Job drawing, mm, ordinate dimensions from the low corner. One solid piece. A direction names the side the tool comes from. Give positions to 0.01 mm unless a question says otherwise; leave off trailing zeros. Order: outer loops, then holes, each group sorted by start corner. A loop starts at its lowest first (then second) coordinate and runs counter-clockwise, first axis right, second up.
1. Drop flat-ended pins along their axis: pin 1 Ø3 at (x, y) = (8.5, 8.5) entering from -Z; pin 2 Ø3 at (y, z) = (15, 0.5) entering from +X; pin 3 Ø1.5 at (x, z) = (13, 0.5) entering from -Y. Give the stop position or say it passes through.
2. Probe line 1 (Y direction, x = 8.5, z = 1.25); line 2 (Z direction, x = 8.25, y = 2.75); line 3 (X direction, y = 7.75, z = 2.05). List the from-to ranges inside material, lowest first.
3. Mould opens along Y. For the marked faces 3, 4 and 5 say: +Y half, -Y half, draft (parallel to the pull), parting line (faces both ways), or undercut.
4. Which spindle directions (+Z, -Z, +X, -X, +Y, -Y) get a long thin tool onto all of the face, cutting with end or side? Do the marked faces 1 and 2. Say none if no direction does.
5. Slice it at D-D on x = 3. List the corners of the cut face in (y, z), and give its area (3 significant figures).
6. Slice it at A-A on y = 8.5. List the corners of the cut face in (x, z), and give its area (3 significant figures).
7. Slice it at C-C on y = 11.5. List the corners of the cut face in (x, z), and give its area (3 significant figures).
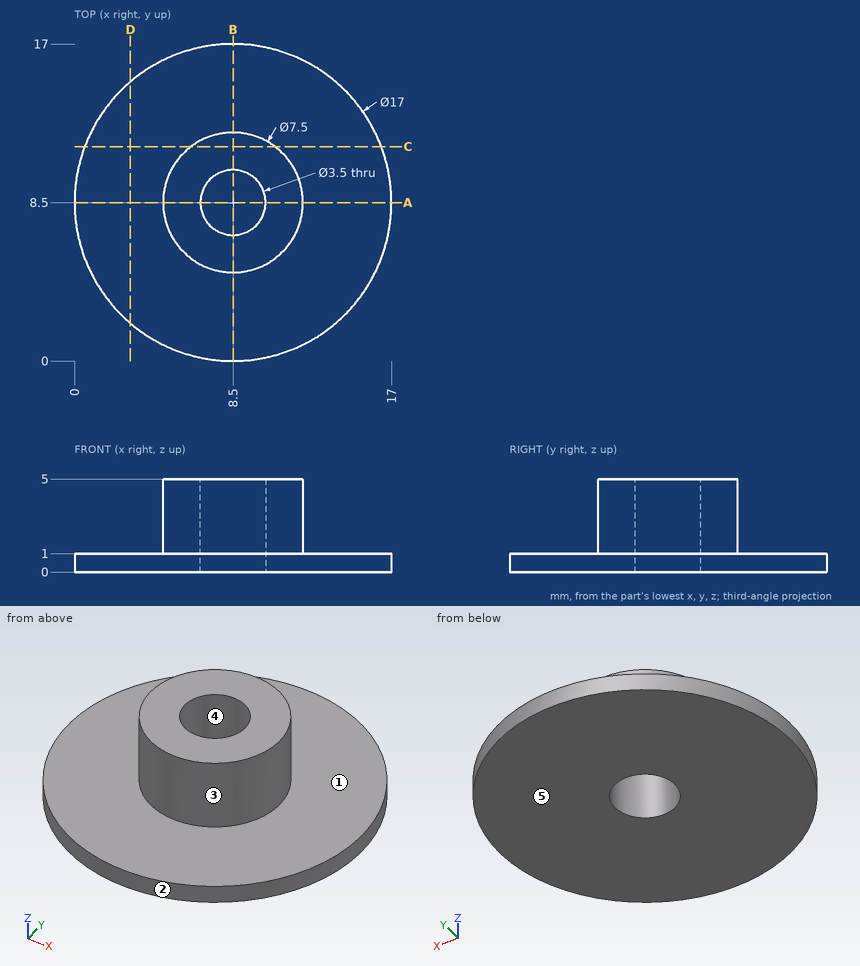
Data:
1. pin 1: passes through
1. pin 2: stops at x = 15.37
1. pin 3: stops at y = 0.87
2. line 1: y = 4.75 to 6.75, 10.25 to 12.25
2. line 2: z = 0 to 1
2. line 3: x = 4.83 to 6.92, 10.08 to 12.17
3. face 3: parting line
3. face 4: undercut
3. face 5: draft
4. face 1: +Z
4. face 2: +Z, -Z
5. outline: (2.02, 0) - (14.98, 0) - (14.98, 1) - (2.02, 1) - close
5. area: 13.0 mm2
6. outline: (0, 0) - (6.75, 0) - (6.75, 5) - (4.75, 5) - (4.75, 1) - (0, 1) - close; (10.25, 0) - (17, 0) - (17, 1) - (12.25, 1) - (12.25, 5) - (10.25, 5) - close
6. area: 29.5 mm2
7. outline: (0.55, 0) - (16.45, 0) - (16.45, 1) - (10.75, 1) - (10.75, 5) - (6.25, 5) - (6.25, 1) - (0.55, 1) - close
7. area: 33.9 mm2
